from build123d import *

# Parameters (mm, degrees)
F0_W      = 95
F0_H      = 50
F0_R      = 2.5
F1_DEPTH  = 10
F2_R      = 12.5
F2_R_2    = 2.5
F3_DEPTH  = 70
F3_FACE_R = 2.5
F4_DEPTH  = 100
F5_SIZE   = 1


with BuildPart() as f1:
    # F0 (on Top) → F1 (new body)
    with BuildSketch(Plane.XY):
        Rectangle(F0_W, F0_H)
        with Locations((-39.5, -17)):
            Circle(F0_R, mode=Mode.SUBTRACT)
        with Locations((39.5, -17)):
            Circle(F0_R, mode=Mode.SUBTRACT)
        with Locations((-39.5, 17)):
            Circle(F0_R, mode=Mode.SUBTRACT)
        with Locations((39.5, 17)):
            Circle(F0_R, mode=Mode.SUBTRACT)
    extrude(amount=F1_DEPTH)

    # F2 (on Top) → F3 (join)
    with BuildSketch(Plane.XY):
        Circle(F2_R)
        Circle(F2_R_2, mode=Mode.SUBTRACT)
    extrude(amount=F3_DEPTH)

    # F3_face (on face) → F4 (cut)
    with BuildSketch(Plane.XY.offset(10)):
        Circle(F3_FACE_R)
    extrude(amount=-F4_DEPTH, mode=Mode.SUBTRACT)

    # F5
    f5_edges = [f1.edges().sort_by_distance(p)[0] for p in [
        (-12.5, 0, 70),
        (-12.5, 0, 10),
    ]]
    chamfer(f5_edges, length=F5_SIZE)


solid = f1.part
The model under review builds one solid part; all positions refer to its coordinate system, in mm. A direction names the side the tool comes from. Round coordinates to 2 decimals unless told otherwise and drop trailing zeros. Write each loop counter-clockwise with the first axis right and the second up, starting at its lowest first coordinate (ties: lowest second). Pieces come first, ordered by that corner, then holes. Notation, with made-up numbers: (8.25, 74.25) - (35.25, 74.25) arc R23 cw to (35.25, 96.25) - close; hole circle Ø8 at (6, 7). An arc over 180 degrees is marked (long way). One line per item, written item: value. Start each with the question number.
1. To check wall thickness, follow L1, parallel to Y at x = -39.5, z = 4; L2, parallel to Y at x = -39, z = 3; L3, parallel to Z at x = 42, y = 10.5. State the ranges of each line that lie inside material, in increasing order. Write a range as from..to.
2. Consider section A-A on x = 39.5. Write out the cut boundary in (y, z).
3. The part is to be moulded in two halves that separate along X. For faces 1 (the face through (-47.5, 0, 5)), 2 (the face through (47.5, 0, 5)), 3 (the face through (-37.19, -17.96, 4.93)), 4 (the face through (-11, 11, 10)), say which applies: released by +X, released by -X, zero draft, split by the parting line, or undercut.
4. Consider section C-C on y = 0. Write out the cut boundary in (x, z), and give its area (3 significant figures).
5. Consider section D-D on z = 8. Write out the cut boundary in (x, y), and give its area (3 significant figures).
6. Clearance check with flat-ended pins moving along their axes: P1, Ø6, axis at x = -39.5, y = 17, coming from the +Z side; P2, Ø2, axis at y = -11.5, z = 39, coming from the -X side; P3, Ø12, axis at y = 6, z = 59.5, coming from the -X side. State where each tip first meets the part, or that it passes through.
7. Machinability: for faces 5 (the face through (41.885, 17.751, 4.93)), 6 (the face through (11.923, 3.755, 39.594)), which of the approach directions +Z, -Z, +X, -X, +Y, -Y give a long, thin tool a straight path to every point of the face, cutting with its end or side? Answer none if there is none.
8. Consider section B-B on x = 0. Write out the cut boundary in (y, z), and give its area (3 significant figures).
Checks:
1. L1: y = -25..-19.5, -14.5..14.5, 19.5..25
1. L2: y = -25..-19.45, -14.55..14.55, 19.45..25
1. L3: z = 0..10
2. outline: (-25, 0) - (-19.5, 0) - (-19.5, 10) - (-25, 10) - close; (-14.5, 0) - (14.5, 0) - (14.5, 10) - (-14.5, 10) - close; (19.5, 0) - (25, 0) - (25, 10) - (19.5, 10) - close
3. face 1: released by -X
3. face 2: released by +X
3. face 3: undercut
3. face 4: zero draft
4. outline: (-47.5, 0) - (-2.5, 0) - (-2.5, 70) - (-11.5, 70) - (-12.5, 69) - (-12.5, 11) - (-13.5, 10) - (-47.5, 10) - close; (2.5, 0) - (47.5, 0) - (47.5, 10) - (13.5, 10) - (12.5, 11) - (12.5, 69) - (11.5, 70) - (2.5, 70) - close
4. area: 2,100 mm^2
5. outline: (-47.5, -25) - (47.5, -25) - (47.5, 25) - (-47.5, 25) - close; hole circle Ø5 at (-39.5, -17); hole circle Ø5 at (-39.5, 17); hole circle Ø5 at (0, 0); hole circle Ø5 at (39.5, -17); hole circle Ø5 at (39.5, 17)
5. area: 4,650 mm^2
6. P1: stops at z = 10
6. P2: stops at x = -6.78
6. P3: stops at x = -12.5
7. face 5: +Z, -Z
7. face 6: +Z
8. outline: (-25, 0) - (-2.5, 0) - (-2.5, 70) - (-11.5, 70) - (-12.5, 69) - (-12.5, 11) - (-13.5, 10) - (-25, 10) - close; (2.5, 0) - (25, 0) - (25, 10) - (13.5, 10) - (12.5, 11) - (12.5, 69) - (11.5, 70) - (2.5, 70) - close
8. area: 1,650 mm^2
